The listing builds one solid part. Answer for the finished solid, in the listing's coordinates (mm). A direction names the side the tool comes from. Coordinates: 2 decimals unless noted, no trailing zeros. Order: outer loops, then holes, each group sorted by start corner. A loop starts at its lowest first (then second) coordinate and runs counter-clockwise, first axis right, second up. Notation, with made-up numbers: (79.25, -23.75) - (89.25, -23.75) arc R16 cw to (89.25, -16.75) - close; hole circle Ø2 at (80.5, 63). An arc over 180 degrees is marked (long way). One line per item, written item: value. Start each with the question number.
```python
from build123d import *

# Parameters (mm, degrees)
SKETCH1_W           = 25.9
SKETCH1_H           = 20
CUT_EXTRUDE1_START  = -6.9
CUT_EXTRUDE1_DEPTH  = 6.9
CUT_EXTRUDE3_DEPTH  = 37.9
CUT_EXTRUDE4_START  = -4
CUT_EXTRUDE4_DEPTH  = 4
SKETCH5_W           = 3.079292118
SKETCH5_H           = 1.929571357
SKETCH5_H_2         = 4.46
SKETCH5_W_2         = 3.459055715
CUT_EXTRUDE5_DEPTH  = 6.9
CUT_EXTRUDE6_START  = -4
SKETCH6_W           = 1.774907729
SKETCH6_H           = 5.455649351
CUT_EXTRUDE6_DEPTH  = 4
SKETCH7_R           = 20.5
BOSS_EXTRUDE1_DEPTH = 0.5
SKETCH8_W           = 5.450728154
SKETCH8_H           = 14.349876159
CUT_EXTRUDE7_DEPTH  = 4
SKETCH9_W           = 5.450728154
SKETCH9_H           = 14.349876159
SKETCH9_W_2         = 4.355367047
SKETCH9_H_2         = 13.330062778
BOSS_EXTRUDE2_DEPTH = 3
SKETCH10_R          = 0.25
BOSS_EXTRUDE3_DEPTH = 3
FILLET1_R           = 0.1
FILLET2_R           = 0.1
FILLET3_R           = 0.1
FILLET4_R           = 0.1
SKETCH11_W          = 9.973758266
SKETCH11_H          = 8.809863574
CUT_EXTRUDE8_DEPTH  = 6.964735979
SKETCH12_W          = 9.973758266
SKETCH12_H          = 8.809863574
SKETCH12_W_2        = 4
SKETCH12_H_2        = 3
BOSS_EXTRUDE4_DEPTH = 6
SKETCH14_R          = 1
CUT_EXTRUDE9_DEPTH  = 12


with BuildPart() as part:
    # Sketch1 → Revolve1 (revolve)
    with BuildSketch(Plane.XY, mode=Mode.PRIVATE) as revolve1_sk:
        with Locations((40.726102109, -10)):
            Rectangle(SKETCH1_W, SKETCH1_H)
    revolve(revolve1_sk.sketch.rotate(Axis((71.094105119, 0, 0), (-1, 0, 0)), 180), axis=Axis((71.094105119, 0, 0), (-1, 0, 0)))

    # Sketch2 → Cut-Extrude1 (cut)
    with BuildSketch(Plane.ZY.offset(-27.776102109).offset(CUT_EXTRUDE1_START)):
        with BuildLine():
            ThreePointArc((7.621425239, 18.490913372), (0.204527107, 19.998954189), (-7.241661642, 18.642916528))
            Line((-7.241661642, 18.642916528), (7.621425239, 18.490913372))
        make_face()
        with BuildLine():
            Line((-7.241661642, 13.035264021), (-7.241661642, 18.642916528))
            ThreePointArc((-7.241661642, 18.642916528), (-11.295281474, -16.50504821), (20, 0))
            ThreePointArc((20, 0), (16.619694714, 11.12590435), (7.621425239, 18.490913372))
            Line((7.621425239, 18.490913372), (7.621425239, 13.035264021))
            Line((7.621425239, 13.035264021), (-7.241661642, 13.035264021))
        make_face()
    extrude(amount=CUT_EXTRUDE1_DEPTH, mode=Mode.SUBTRACT)

    # Sketch3 → Cut-Extrude3 (cut)
    with BuildSketch(Plane.XY.offset(7.621425239)):
        Polygon((27.776102109, 17.495264021), (34.676102109, 18.490913372), (27.776102109, 18.490913372), align=None)
        Polygon((27.776102109, 18.490913372), (34.676102109, 18.490913372), (34.676102109, 18.667614819), (27.776102109, 19.075412015), align=None)
    extrude(amount=-CUT_EXTRUDE3_DEPTH, mode=Mode.SUBTRACT)

    # Sketch4 → Cut-Extrude4 (cut)
    with BuildSketch(Plane.ZY.offset(-34.676102109).offset(CUT_EXTRUDE4_START)):
        with BuildLine():
            ThreePointArc((5.466753913, 5.13464718), (0, -7.5), (-5.466753913, 5.13464718))
            Line((-5.466753913, 5.13464718), (-5.466753913, 13.035264021))
            Line((-5.466753913, 13.035264021), (-7.241661642, 13.035264021))
            Line((-7.241661642, 13.035264021), (-7.241661642, 18.490913372))
            Line((-7.241661642, 18.490913372), (-5.466753913, 18.490913372))
            Line((-5.466753913, 18.490913372), (-5.466753913, 19.238362759))
            ThreePointArc((-5.466753913, 19.238362759), (-12.055391361, -15.958306274), (20, 0))
            ThreePointArc((20, 0), (16.619694714, 11.12590435), (7.621425239, 18.490913372))
            Line((7.621425239, 18.490913372), (7.621425239, 13.035264021))
            Line((7.621425239, 13.035264021), (5.466753913, 13.035264021))
            Line((5.466753913, 13.035264021), (5.466753913, 5.13464718))
        make_face()
    extrude(amount=CUT_EXTRUDE4_DEPTH, mode=Mode.SUBTRACT)

    # Sketch5 → Cut-Extrude5 (cut)
    with BuildSketch(Plane.ZY.offset(-27.776102109)):
        with Locations((-5.702015583, 18.4600497)):
            Rectangle(SKETCH5_W, SKETCH5_H)
        with Locations((-5.702015583, 15.265264021)):
            Rectangle(SKETCH5_W, SKETCH5_H_2)
        with Locations((5.891897381, 18.4600497)):
            Rectangle(SKETCH5_W_2, SKETCH5_H)
        with Locations((5.891897381, 15.265264021)):
            Rectangle(SKETCH5_W_2, SKETCH5_H_2)
    extrude(amount=-CUT_EXTRUDE5_DEPTH, mode=Mode.SUBTRACT)

    # Sketch6 → Cut-Extrude6 (cut)
    with BuildSketch(Plane.ZY.offset(-34.676102109).offset(CUT_EXTRUDE6_START)):
        with BuildLine():
            Line((5.466753913, 19.238362759), (5.466753913, 13.035264021))
            Line((5.466753913, 13.035264021), (7.621425239, 13.035264021))
            Line((7.621425239, 13.035264021), (7.621425239, 18.490913372))
            ThreePointArc((7.621425239, 18.490913372), (6.554752362, 18.895375664), (5.466753913, 19.238362759))
        make_face()
        with Locations((-6.354207778, 15.763088697)):
            Rectangle(SKETCH6_W, SKETCH6_H)
    extrude(amount=CUT_EXTRUDE6_DEPTH, mode=Mode.SUBTRACT)

    # Sketch7 → Boss-Extrude1 (add, symmetric)
    with BuildSketch(Plane.ZY.offset(-46.176102109)):
        with Locations(Location((0, 0, 0), (0, 0, 270))):
            Circle(SKETCH7_R)
    extrude(amount=BOSS_EXTRUDE1_DEPTH, both=True)

    # Sketch8 → Cut-Extrude7 (cut)
    with BuildSketch(Plane.ZY.offset(-38.676102109)):
        with Locations((-15.184171285, 0.083429512)):
            Rectangle(SKETCH8_W, SKETCH8_H)
    extrude(amount=-CUT_EXTRUDE7_DEPTH, mode=Mode.SUBTRACT)

    # Sketch9 → Boss-Extrude2 (add)
    with BuildSketch(Plane.ZY.offset(-42.676102109)):
        with Locations((-15.184171285, 0.083429512)):
            Rectangle(SKETCH9_W, SKETCH9_H)
        with Locations((-15.184204235, 0.116814581)):
            Rectangle(SKETCH9_W_2, SKETCH9_H_2, mode=Mode.SUBTRACT)
    extrude(amount=BOSS_EXTRUDE2_DEPTH)

    # Sketch10 → Boss-Extrude3 (add)
    with BuildSketch(Plane.ZY.offset(-42.676102109)):
        with Locations((-15.826659994, 4.106898055)):
            Circle(SKETCH10_R)
        with Locations((-15.826659994, 1.606898055)):
            Circle(SKETCH10_R)
        with Locations((-15.826659994, -3.393101945)):
            Circle(SKETCH10_R)
        with Locations((-15.826659994, -0.893101945)):
            Circle(SKETCH10_R)
    extrude(amount=BOSS_EXTRUDE3_DEPTH)

    # Fillet1
    fillet1_edges = [part.edges().sort_by_distance(p)[0] for p in [
        (39.676102109, 4.106898055, -16.076659994),
    ]]
    fillet(fillet1_edges, radius=FILLET1_R)

    # Fillet2
    fillet2_edges = [part.edges().sort_by_distance(p)[0] for p in [
        (39.676102109, 1.606898055, -16.076659994),
    ]]
    fillet(fillet2_edges, radius=FILLET2_R)

    # Fillet3
    fillet3_edges = [part.edges().sort_by_distance(p)[0] for p in [
        (39.676102109, -0.893101945, -16.076659994),
    ]]
    fillet(fillet3_edges, radius=FILLET3_R)

    # Fillet4
    fillet4_edges = [part.edges().sort_by_distance(p)[0] for p in [
        (39.676102109, -3.393101945, -16.076659994),
    ]]
    fillet(fillet4_edges, radius=FILLET4_R)

    # Sketch11 → Cut-Extrude8 (cut)
    with BuildSketch(Plane(origin=(0, 20, 0), x_dir=(1, 0, 0), z_dir=(0, 1, 0))):
        with Locations((40.689222976, 0.086069267)):
            Rectangle(SKETCH11_W, SKETCH11_H)
    extrude(amount=-CUT_EXTRUDE8_DEPTH, mode=Mode.SUBTRACT)

    # Sketch12 → Boss-Extrude4 (add)
    with BuildSketch(Plane(origin=(0, 13.035264021, 0), x_dir=(1, 0, 0), z_dir=(0, 1, 0))):
        with Locations((40.689222976, 0.086069267)):
            Rectangle(SKETCH12_W, SKETCH12_H)
        with Locations((38.421750687, -1.928820044)):
            Rectangle(SKETCH12_W_2, SKETCH12_H_2, mode=Mode.SUBTRACT)
        with Locations((38.366922829, 2.435416113)):
            Rectangle(SKETCH12_W_2, SKETCH12_H_2, mode=Mode.SUBTRACT)
    extrude(amount=BOSS_EXTRUDE4_DEPTH)

    # Sketch14 → Cut-Extrude9 (cut)
    with BuildSketch(Plane(origin=(36.421750687, 0, 0), x_dir=(0, 0, -1), z_dir=(1, 0, 0))):
        with Locations(Location((-1.928820044, 16.035264021, 0), (0, 0, 90))):
            Circle(SKETCH14_R)
        with Locations(Location((2.105292071, 16.035264021, 0), (0, 0, 90))):
            Circle(SKETCH14_R)
    extrude(amount=-CUT_EXTRUDE9_DEPTH, mode=Mode.SUBTRACT)


solid = part.part
```
(1) For a pull along Z with two mould halves and no side action, classify faces 4 (the face through (38, 16, 0.429)), 5 (the face through (37, 12, -5.467)), 6 (the face through (31, 16, 4.162)), 7 (the face through (34.676, 6, 0)) as pulls with the +Z half, pulls with the -Z half, needs draft (parallel to the pull), parting line crosses it, or undercut.
(2) The part is cut by section C-C on x = 49. Determine the outline of the cut face in (y, z), plus the area to 3 significant figures.
(3) For faces 1 (the face through (39, 0, -12.459)), 2 (the face through (36.422, 17, 3)), 3 (the face through (50.23, -19.98, -0.88)), determine the directions among +Z, -Z, +X, -X, +Y, -Y from which every point of the face is accessible in a straight line to the end or side of a thin tool.
(4) Consider probe 1 along X at (y, z) = (9, -17.5); probe 2 along Z at (x, y) = (35.25, 17.5); probe 3 along Z at (x, y) = (39.5, 2.5). Determine where each line is inside the solid, lowest interval first.
(5) The part is cut by section D-D on x = 33. Determine the outline of the cut face in (y, z).
(6) Flat-ended cylindrical pins translate along their axes: pin 1 Ø0.9 at (x, z) = (39, -3) entering from +Y; pin 2 Ø1.1 at (x, z) = (39.5, -15.5) entering from +Y; pin 3 Ø4.5 at (x, y) = (37, 9.5) entering from -Z. Find the tip coordinate at first contact, or state that the pin passes through.
(7) The part is cut by section B-B on z = 18. Determine the outline of the cut face in (x, y).
(8) The part is cut by section A-A on y = 0. Determine the outline of the cut face in (x, z).
Completed:
1. face 4: undercut
1. face 5: pulls with the -Z half
1. face 6: pulls with the +Z half
1. face 7: needs draft
2. outline: circle Ø40 at (0, 0)
2. area: 1,260 mm2
3. face 1: -X
3. face 2: +Y
3. face 3: +X
4. probe 1: x = 38.68 to 53.68
4. probe 2: z = -5.47 to 5.47
4. probe 3: z = -19.84 to -17.91, -12.46 to 19.84
5. outline: (13.04, -4.16) - (18.25, -4.16) - (18.25, 4.16) - (13.04, 4.16) - close; hole circle Ø2 at (16.04, -2.11); hole circle Ø2 at (16.04, 1.93)
6. pin 1: stops at y = 13.04
6. pin 2: stops at y = 13.29
6. pin 3: stops at z = -18.33
7. outline: (38.68, -8.72) - (45.68, -8.72) - (45.68, -9.81) - (46.68, -9.81) - (46.68, -8.72) - (53.68, -8.72) - (53.68, 8.72) - (46.68, 8.72) - (46.68, 9.81) - (45.68, 9.81) - (45.68, 8.72) - (38.68, 8.72) - close
8. outline: (34.68, -7.5) - (38.68, -7.5) - (38.68, -12.46) - (39.68, -12.46) - (39.68, -13.01) - (42.68, -13.01) - (42.68, -17.36) - (39.68, -17.36) - (39.68, -17.91) - (38.68, -17.91) - (38.68, -20) - (45.68, -20) - (45.68, -20.5) - (46.68, -20.5) - (46.68, -20) - (53.68, -20) - (53.68, 20) - (46.68, 20) - (46.68, 20.5) - (45.68, 20.5) - (45.68, 20) - (38.68, 20) - (38.68, 7.5) - (34.68, 7.5) - close
